Can you work these out from the model? Positions are in its coordinate system, mm. A direction names the side the tool comes from. Coordinates: 2 decimals unless noted, no trailing zeros. Loops run counter-clockwise (first coordinate to the right, second up) from the corner with the lowest first, then second, coordinate; pieces in that order, holes last. Notation, with made-up numbers: (24.25, 79.5) - (53.25, 79.5) arc R19 cw to (53.25, 88.5) - close; hole circle Ø10 at (11, -23.5). An arc over 180 degrees is marked (long way). Put each result on its own line as item: value. Start each with the question number.
from build123d import *

# Parameters (mm, degrees)
BOSS_EXTRUDE1_DEPTH = 20
FILLET1_R           = 2.5
CUT_EXTRUDE1_REACH  = 183.384
SKETCH4_R           = 10
BOSS_EXTRUDE2_DEPTH = 20
SKETCH5_R           = 15
BOSS_EXTRUDE3_DEPTH = 5
FILLET2_R           = 2.5


with BuildPart() as part:
    # Sketch1 → Boss-Extrude1 (new body)
    with BuildSketch(Plane(origin=(0, 0, 0), x_dir=(1, 0, 0), z_dir=(0, 1, 0))):
        with BuildLine():
            Line((-140, 100), (140, 100))
            ThreePointArc((140, 100), (147.071067812, 97.071067812), (150, 90))
            Line((150, 90), (150, -90))
            ThreePointArc((150, -90), (147.071067812, -97.071067812), (140, -100))
            Line((140, -100), (-140, -100))
            ThreePointArc((-140, -100), (-147.071067812, -97.071067812), (-150, -90))
            Line((-150, -90), (-150, 90))
            ThreePointArc((-150, 90), (-147.071067812, 97.071067812), (-140, 100))
        make_face()
    extrude(amount=BOSS_EXTRUDE1_DEPTH)

    # Fillet1
    fillet1_edges = [part.edges().sort_by_distance(p)[0] for p in [
        (-147.071067812, 20, -97.071067812),
        (-150, 20, 0),
        (-147.071067812, 20, 97.071067812),
        (0, 20, 100),
        (147.071067812, 20, 97.071067812),
        (150, 20, 0),
        (147.071067812, 20, -97.071067812),
        (0, 20, -100),
    ]]
    fillet(fillet1_edges, radius=FILLET1_R)

    # Sketch3 → Cut-Extrude1 (cut, up to next)
    with BuildSketch(Plane(origin=(0, 20, 0), x_dir=(1, 0, 0), z_dir=(0, 1, 0)), mode=Mode.PRIVATE) as cut_extrude1_sk1:
        with BuildLine():
            Line((-122.5, -75), (-122.5, 60))
            ThreePointArc((-122.5, 60), (-120.303300859, 65.303300859), (-115, 67.5))
            Line((-115, 67.5), (15, 67.5))
            ThreePointArc((15, 67.5), (20.303300859, 65.303300859), (22.5, 60))
            Line((22.5, 60), (22.5, 15))
            ThreePointArc((22.5, 15), (29.090097423, -0.909902577), (45, -7.5))
            Line((45, -7.5), (110, -7.5))
            ThreePointArc((110, -7.5), (115.303300859, -9.696699141), (117.5, -15))
            Line((117.5, -15), (117.5, -75))
            ThreePointArc((117.5, -75), (125, -82.5), (132.5, -75))
            Line((132.5, -75), (132.5, -15))
            ThreePointArc((132.5, -15), (125.909902577, 0.909902577), (110, 7.5))
            Line((110, 7.5), (45, 7.5))
            ThreePointArc((45, 7.5), (39.696699141, 9.696699141), (37.5, 15))
            Line((37.5, 15), (37.5, 60))
            ThreePointArc((37.5, 60), (30.909902577, 75.909902577), (15, 82.5))
            Line((15, 82.5), (-115, 82.5))
            ThreePointArc((-115, 82.5), (-130.909902577, 75.909902577), (-137.5, 60))
            Line((-137.5, 60), (-137.5, -75))
            ThreePointArc((-137.5, -75), (-130, -82.5), (-122.5, -75))
        make_face()
    cut_extrude1_tool1 = extrude(cut_extrude1_sk1.sketch, amount=-CUT_EXTRUDE1_REACH, mode=Mode.PRIVATE) & part.part
    add(cut_extrude1_tool1.solids().sort_by_distance((-125.664253, 20, 7.5))[0], mode=Mode.SUBTRACT)

    # Sketch4 → Boss-Extrude2 (add)
    with BuildSketch(Plane(origin=(0, 20, 0), x_dir=(1, 0, 0), z_dir=(0, 1, 0))):
        with Locations(Location((-30, -70, 0), (0, 0, 90))):
            Circle(SKETCH4_R)
    extrude(amount=BOSS_EXTRUDE2_DEPTH)

    # Sketch5 → Boss-Extrude3 (add)
    with BuildSketch(Plane(origin=(0, 40, 0), x_dir=(1, 0, 0), z_dir=(0, 1, 0))):
        with Locations(Location((-30, -70, 0), (0, 0, 270))):
            Circle(SKETCH5_R)
    extrude(amount=BOSS_EXTRUDE3_DEPTH)

    # Fillet2
    fillet2_edges = [part.edges().sort_by_distance(p)[0] for p in [
        (-30, 45, 55),
    ]]
    fillet(fillet2_edges, radius=FILLET2_R)


solid = part.part
Q1. Will this pin go through, and if not, where does the flat tip stop? pin 1 (3 mm diameter, centred on x = 84.5, z = -34, fed in from +Y).
Q2. I want a section at B-B on z = 70. List the corners of the cut face in (x, y) for me, and give its area (3 significant figures).
Q3. I want a section at D-D on z = -77. List the corners of the cut face in (x, y) for me, and give its area (3 significant figures).
Q4. I want a section at A-A on x = 85.5. List the corners of the cut face in (y, z) for me, and give its area (3 significant figures).
Q5. We'd pull the mould along Y, two halves only. Please class faces 1 (the flat face through (-30, 45, 70)), 2 (the flat face through (-33, 40, 80)), 3 (the flat face through (150, 9, -1)): released by +Y, released by -Y, zero draft, split by the parting line, or undercut.
Q6. I want a section at C-C on y = 7. List the corners of the cut face in (x, z) for me.
Q7. On a 3-axis mill with a long thin cutter (end or side, diameter ignored), from which of +Z, -Z, +X, -X, +Y, -Y can I reach the whole of each face in a straight line? I mean faces 4 (the flat face through (2, 9, 100)), 5 (the cylindrical face through (124.84, 10.14, 82.5)). Say none if no direction works.
Q8. Please list where these lines run through material, in increasing order: line 1 along X through (y, z) = (8, 51.5); line 2 along X through (y, z) = (7, -12); line 3 along Y through (x, z) = (68.5, 14). Write a range as [from, to].
Calculated:
1. pin 1: y = 20
2. outline: (-150, 0) - (-137.5, 0) - (-137.5, 20) - (-147.5, 20) arc R2.5 ccw to (-150, 17.5) - close; (-122.5, 0) - (117.5, 0) - (117.5, 20) - (-20, 20) - (-20, 40) - (-15, 40) - (-15, 42.5) arc R2.5 ccw to (-17.5, 45) - (-42.5, 45) arc R2.5 ccw to (-45, 42.5) - (-45, 40) - (-40, 40) - (-40, 20) - (-122.5, 20) - close; (132.5, 0) - (150, 0) - (150, 17.5) arc R2.5 ccw to (147.5, 20) - (132.5, 20) - close
2. area: 5,940 mm2
3. outline: (-150, 0) - (-129.74, 0) - (-129.74, 20) - (-147.5, 20) arc R2.5 ccw to (-150, 17.5) - close; (29.74, 0) - (150, 0) - (150, 17.5) arc R2.5 ccw to (147.5, 20) - (29.74, 20) - close
3. area: 2,810 mm2
4. outline: (0, -100) - (17.5, -100) arc R2.5 ccw to (20, -97.5) - (20, -7.5) - (0, -7.5) - close; (0, 7.5) - (20, 7.5) - (20, 97.5) arc R2.5 ccw to (17.5, 100) - (0, 100) - close
4. area: 3,700 mm2
5. face 1: released by +Y
5. face 2: undercut
5. face 3: zero draft
6. outline: (-150, -90) arc R10 ccw to (-140, -100) - (140, -100) arc R10 ccw to (150, -90) - (150, 90) arc R10 ccw to (140, 100) - (-140, 100) arc R10 ccw to (-150, 90) - close; hole (-137.5, -60) arc R22.5 ccw to (-115, -82.5) - (15, -82.5) arc R22.5 ccw to (37.5, -60) - (37.5, -15) arc R7.5 cw to (45, -7.5) - (110, -7.5) arc R22.5 ccw to (132.5, 15) - (132.5, 75) arc R7.5 ccw to (117.5, 75) - (117.5, 15) arc R7.5 cw to (110, 7.5) - (45, 7.5) arc R22.5 ccw to (22.5, -15) - (22.5, -60) arc R7.5 cw to (15, -67.5) - (-115, -67.5) arc R7.5 cw to (-122.5, -60) - (-122.5, 75) arc R7.5 ccw to (-137.5, 75) - close
7. face 4: +Z, +X, -X, +Y, -Y
7. face 5: +Y, -Y
8. line 1: [-150, -137.5], [-122.5, 117.5], [132.5, 150]
8. line 2: [-150, -137.5], [-122.5, 22.7], [38.13, 150]
8. line 3: [0, 20]
